```python
from build123d import *

# Parameters (mm, degrees)
F0_W     = 96.52
F0_H     = 15.24
F1_DEPTH = 5.588
F2_W     = 7.62
F2_H     = 6.35
F3_DEPTH = 25.4
F4_R     = 2.54


with BuildPart() as f1:
    # F0 (on Front) → F1 (new body)
    with BuildSketch(Plane.XZ):
        with Locations((48.26, -7.62)):
            Rectangle(F0_W, F0_H)
    extrude(amount=F1_DEPTH)

    # F2 (on face) → F3 (cut)
    with BuildSketch(Plane.XZ.offset(5.588)):
        with Locations((92.71, -12.065)):
            Rectangle(F2_W, F2_H)
        with Locations((3.81, -12.065)):
            Rectangle(F2_W, F2_H)
    extrude(amount=-F3_DEPTH, mode=Mode.SUBTRACT)

    # F4
    f4_edges = [f1.edges().sort_by_distance(p)[0] for p in [
        (48.26, 0, 0),
        (48.26, -5.588, 0),
    ]]
    fillet(f4_edges, radius=F4_R)


solid = f1.part
```
Check sheet for the modelled part. Datum: model origin and axes. Units: mm. A direction names the side the tool comes from. Give positions to 0.01 mm unless a question says otherwise; leave off trailing zeros. Order: outer loops, then holes, each group sorted by start corner. A loop starts at its lowest first (then second) coordinate and runs counter-clockwise, first axis right, second up. Notation, with made-up numbers: (24.25, -6.75) -> (80.25, -6.75) arc R23 ccw to (80.25, 3.25) -> close; hole circle Ø8 at (-37.75, 52.5). An arc over 180 degrees is marked (long way). Use CSV: the item, a comma, the result in double quotes. Start each with the question number.
1) Sectioned sample at A-A, the plane x = 31. Record the boundary of the cut face in (y, z), plus the area to 3 significant figures.
2) Material ranges on line 1 (X direction, y = -3.95, z = -10.75); line 2 (Y direction, x = 57.5, z = -2.25); line 3 (Z direction, x = 15, y = -3.3), recorded low to high. Write a range as from..to.
3) Set-up check for faces 1 (the face through (7.62, -3, -12)), 2 (the face through (88.9, -3, -12)), 3 (the face through (0, -3, -5)): record each of +Z, -Z, +X, -X, +Y, -Y from which the full face is reachable in a straight line by a thin tool's end or side.
4) Sectioned sample at D-D, the plane z = -1.75. Record the boundary of the cut face in (x, y), plus the area to 3 significant figures.
5) Sectioned sample at B-B, the plane y = -1.15. Record the boundary of the cut face in (x, z).
6) Go/stop test with flat-tipped pins: P1, Ø3, axis at x = 3.5, y = -3, coming from the -Z side; P2, Ø3, axis at y = -2, z = -11.5, coming from the +X side; P3, Ø1.7, axis at y = -3.5, z = -13, coming from the -X side. Record where each tip stops, or that it passes through.
7) Sectioned sample at C-C, the plane z = -10. Record the boundary of the cut face in (x, y).
Recorded:
1,outline,"(-5.59, -15.24) -> (0, -15.24) -> (0, -2.54) arc R2.54 ccw to (-2.54, 0) -> (-3.05, 0) arc R2.54 ccw to (-5.59, -2.54) -> close"
1,area,"82.4 mm2"
2,line 1,"7.62..88.9"
2,line 2,"-5.57..-0.02"
2,line 3,"-15.24..-0.01"
3,face 1,"-Z, -X, +Y, -Y"
3,face 2,"-Z, +X, +Y, -Y"
3,face 3,"+Z, -Z, -X, +Y, -Y"
4,outline,"(0, -5.46) -> (96.52, -5.46) -> (96.52, -0.13) -> (0, -0.13) -> close"
4,area,"515 mm2"
5,outline,"(0, -8.89) -> (7.62, -8.89) -> (7.62, -15.24) -> (88.9, -15.24) -> (88.9, -8.89) -> (96.52, -8.89) -> (96.52, -0.41) -> (0, -0.41) -> close"
6,P1,"z = -8.89"
6,P2,"x = 88.9"
6,P3,"x = 7.62"
7,outline,"(7.62, -5.59) -> (88.9, -5.59) -> (88.9, 0) -> (7.62, 0) -> close"
